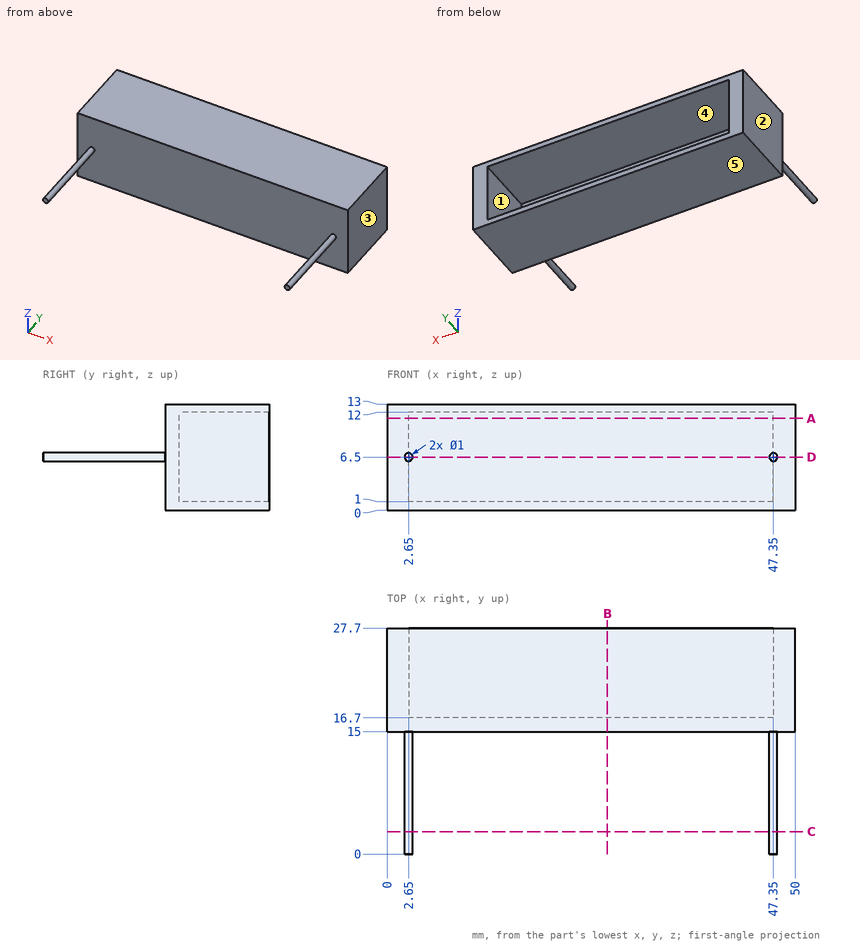
Part print with two shaded views. Sizes in mm from the minimum x, y, z corner. A direction names the side the tool comes from. Give positions to 0.01 mm unless a question says otherwise; leave off trailing zeros. Order: outer loops, then holes, each group sorted by start corner. A loop starts at its lowest first (then second) coordinate and runs counter-clockwise, first axis right, second up.
1) Saw through at A-A, the plane z = 11.25. Write the cut outline in (x, y), then the cut area to 3 significant figures.
2) 3-axis set-ups, long thin cutter, end or side, ignore diameter. For the marked faces 1 and 2: which of +Z, -Z, +X, -X, +Y, -Y reach the whole face in a straight line?
3) Wall check: probe 1 along Z at (x, y) = (29, 19.75); probe 2 along X at (y, z) = (20.5, 6); probe 3 along X at (y, z) = (11, 6.5). Give the ranges that are in metal, low to high.
4) Mould opens along X. For the marked faces 3, 4 and 5 say: +X half, -X half, draft (parallel to the pull), parting line (faces both ways), or undercut.
5) Saw through at C-C, the plane y = 2.75. Write the cut outline in (x, z).
6) Pin check, flat tips, straight feed: pin 1 (5 mm diameter, centred on x = 33.5, z = 2, fed in from -Y); pin 2 (2 mm diameter, centred on x = 41.5, z = 4, fed in from +Y). Stop position of each tip, or through.
7) Saw through at D-D, the plane z = 6.5. Write the cut outline in (x, y).
8) Saw through at B-B, the plane x = 27. Write the cut outline in (y, z).
Computed:
1. outline: (0, 15) - (50, 15) - (50, 27.7) - (47.35, 27.7) - (47.35, 16.7) - (2.65, 16.7) - (2.65, 27.7) - (0, 27.7) - close
1. area: 143 mm2
2. face 1: +Y
2. face 2: +Z, -Z, -X, +Y, -Y
3. probe 1: z = 0 to 1, 12 to 13
3. probe 2: x = 0 to 2.65, 47.35 to 50
3. probe 3: x = 2.15 to 3.15, 46.85 to 47.85
4. face 3: +X half
4. face 4: undercut
4. face 5: draft
5. outline: circle Ø1 at (2.65, 6.5); circle Ø1 at (47.35, 6.5)
6. pin 1: stops at y = 15
6. pin 2: stops at y = 16.7
7. outline: (0, 15) - (2.15, 15) - (2.15, 0) - (3.15, 0) - (3.15, 15) - (46.85, 15) - (46.85, 0) - (47.85, 0) - (47.85, 15) - (50, 15) - (50, 27.7) - (47.35, 27.7) - (47.35, 16.7) - (2.65, 16.7) - (2.65, 27.7) - (0, 27.7) - close
8. outline: (15, 0) - (27.7, 0) - (27.7, 1) - (16.7, 1) - (16.7, 12) - (27.7, 12) - (27.7, 13) - (15, 13) - close
